Autodesk Inventor part; units mm, degrees
ref_plane "YZ Plane" through (0, 0, 0) normal (1, 0, 0) x (0, 1, 0)
ref_plane "XZ Plane" through (0, 0, 0) normal (0, 1, 0) x (-1, 0, 0)
ref_plane "XY Plane" through (0, 0, 0) normal (0, 0, 1) x (1, 0, 0)
sketch "Esquisse1" plane through (0, 0, 0) normal (0, 1, 0) x (-1, 0, 0)
  line L0 (21, 10.5) -> (-21, 10.5)
  line L1 (-21, 10.5) -> (-21, -10.5)
  line L2 (-21, -10.5) -> (21, -10.5)
  line L3 (21, -10.5) -> (21, 10.5)
  line L4 (29, 12.5) -> (-37, 12.5)
  line L5 (-37, 12.5) -> (-37, -12.5)
  line L6 (-37, -12.5) -> (29, -12.5)
  line L7 (29, -12.5) -> (29, 12.5)
  line L8 (-37, -12.5) -> (-46.0993, 12.5)
  line L9 (-46.0993, 12.5) -> (-37, 12.5)
  point P0 (0, 0)
  dimension "d0" = 20
  dimension "d1" = 42
  dimension "d2" = 21
  dimension "d3" = 10.5
  dimension "d4" = 21
  dimension "d5" = 8
  dimension "d6" = 2
  dimension "d7" = 2
  dimension "d8" = 16
extrude "Extrusion1" add sketch "Esquisse1" along normal mid plane 25
sketch "Esquisse2" plane through (37, -12.5, -12.5) normal (0.9397, 0, -0.342) x (-0.342, 0, -0.9397)
  line L0 (-26.6044, 25) -> (0, 0)
  line L1 (0, 0) -> (0, 25)
  line L2 (0, 25) -> (-26.6044, 0)
  arc A0 (-8.3022, 22.298) -> (-18.3022, 22.298) centre (-13.3022, 12.5) ccw
  line L3 (-18.3022, 22.298) -> (-8.3022, 22.298)
  line L4 (-8.3022, 22.298) -> (-8.3022, 2.702)
  line L5 (-8.3022, 2.702) -> (-18.3022, 2.702)
  line L6 (-18.3022, 2.702) -> (-18.3022, 22.298)
  arc A1 (-8.3022, 2.702) -> (-8.3022, 22.298) centre (-13.3022, 12.5) ccw
  arc A2 (-18.3022, 2.702) -> (-8.3022, 2.702) centre (-13.3022, 12.5) ccw
  arc A3 (-18.3022, 22.298) -> (-18.3022, 2.702) centre (-13.3022, 12.5) ccw
  point P0 (0.9086, 12.5)
  point P1 (-26.6044, 25)
  point P2 (-26.6044, 0)
  dimension "d11" = 22
  dimension "d13" = 10
extrude "Extrusion2" add sketch "Esquisse2" along normal blind 5 contours A3 L6 L0 | L0 L6 L2 A3 | L6 L3 L4 L2 L0 | L0 L2 L6 | L2 L6 A3 | L2 L4 L0 | L0 L4 L5 L6 L2 | A1 L2 L4 | L4 L2 A1 L0 | L0 A1 L4
sketch "Esquisse3" plane through (39.8395, -9.798, -4.6985) normal (0, -1, 0) x (0.9397, 0, -0.342)
  line L0 (5, 10) -> (0, 0)
  line L1 (0, 10) -> (5, 0)
  circle A0 centre (2.5, 5) radius 1.75
  point P0 (-39.0439, -9.2108)
  dimension "d16" = 3.5
extrude "Extrusion3" cut sketch "Esquisse3" against normal through all
sketch "Esquisse4" plane through (21, -12.5, 10.5) normal (-1, 0, 0) x (0, 0, 1)
  line L0 (-21, 3) -> (0, 3)
  line L1 (0, 3) -> (0, 6)
  line L2 (0, 6) -> (-21, 6)
  line L3 (-21, 6) -> (-21, 3)
  line L4 (-21, 0) -> (-21, 25)
  line L5 (0, 0) -> (0, 25)
  line L6 (0, 0) -> (-21, 0)
  point P0 (-10.5, 12.5)
  dimension "d19" = 3
  dimension "d20" = 3
extrude "Extrusion4" cut sketch "Esquisse4" against normal blind 7 contours L3 L2 L1 L0
sketch "Esquisse5" plane through (-21, -12.5, -10.5) normal (1, 0, 0) x (0, 0, -1)
  line L0 (-21, 6) -> (0, 6)
  line L1 (0, 6) -> (0, 3)
  line L2 (0, 3) -> (-21, 3)
  line L3 (-21, 3) -> (-21, 6)
  line L4 (-21, 25) -> (-21, 0)
  line L5 (0, 0) -> (0, 25)
  line L6 (0, 0) -> (-21, 0)
  point P0 (-10.5, 12.5)
  dimension "d23" = 3
  dimension "d24" = 3
extrude "Extrusion5" cut sketch "Esquisse5" against normal blind 7 contours L0 L1 L2 L3
sketch "Esquisse6" plane through (21, 12.5, -10.5) normal (-1, 0, 0) x (0, 0, 1)
  line L0 (21, -25) -> (0, 0)
  line L1 (0, -25) -> (21, 0)
  circle A0 centre (10.5, -12.5) radius 3
  dimension "d27" = 6
extrude "Extrusion6" cut sketch "Esquisse6" against normal through all
sketch "Esquisse7" plane through (21, 12.5, -10.5) normal (-1, 0, 0) x (0, 0, 1)
  circle A0 centre (10.5, -12.5) radius 3
  circle A1 centre (10.5, -12.5) radius 1.75
  circle A2 centre (10.5, -12.5) radius 3
  dimension "d30" = 0
  dimension "d31" = 3.5
extrude "Extrusion7" add sketch "Esquisse7" against normal blind 18
sketch "Esquisse8" plane through (21, 12.5, -10.5) normal (-1, 0, 0) x (0, 0, 1)
  circle A0 centre (10.5, -12.5) radius 4
  dimension "d34" = 8
extrude "Extrusion8" cut sketch "Esquisse8" against normal blind 3
sketch "Esquisse10" plane through (0, -12.5, 0) normal (0, -1, 0) x (1, 0, 0)
  line L0 (-21, -10.5) -> (-28, -10.5)
  line L1 (-28, -10.5) -> (-28, 10.5)
  line L2 (-28, 10.5) -> (-21, 10.5)
  line L3 (-21, 10.5) -> (-21, -10.5)
  line L4 (21, -10.5) -> (28, -10.5)
  line L5 (28, -10.5) -> (28, 10.5)
  line L6 (28, 10.5) -> (21, 10.5)
  line L7 (21, 10.5) -> (21, -10.5)
  line L8 (-28, -10.5) -> (-28, 10.5)
  line L9 (28, 10.5) -> (28, -10.5)
  line L10 (-28, -10.5) -> (-21, 0)
  line L11 (-21, 0) -> (-28, 10.5)
  line L12 (-28, 0) -> (-21, 10.5)
  line L13 (-21, -10.5) -> (-28, 0)
  line L14 (21, -10.5) -> (28, 0)
  line L15 (21, 0) -> (28, -10.5)
  line L16 (28, 10.5) -> (21, 0)
  line L17 (21, 10.5) -> (28, 0)
  circle A0 centre (-24.5, -5.25) radius 2
  circle A1 centre (24.5, -5.25) radius 2
  circle A2 centre (24.5, 5.25) radius 2
  circle A3 centre (-24.5, 5.25) radius 2
  point P0 (0, 0)
  dimension "d37" = 4
  dimension "d38" = 4
  dimension "d39" = 4
  dimension "d40" = 4
extrude "Extrusion9" cut sketch "Esquisse10" against normal through all contours A0 L10 L13 | L13 L10 A0 | A0 L13 L10 | L10 L13 A0 | A3 L12 L11 | L11 L12 A3 | A3 L11 L12 | L12 L11 A3 | A1 L15 L14 | L14 L15 A1 | L15 L14 A1 | A1 L14 L15 | A2 L17 L16 | L16 L17 A2 | L17 L16 A2 | A2 L16 L17
sketch "Esquisse11" plane through (37, 12.5, -12.5) normal (0, 0, -1) x (-1, 0, 0)
  line L0 (66, 0) -> (46, 0)
  line L1 (46, 0) -> (46, -13)
  line L2 (46, -13) -> (66, -13)
  line L3 (66, -13) -> (66, 0)
  line L4 (66, -25) -> (0, -25)
  line L5 (46, -13) -> (33, 0)
  line L6 (0, 0) -> (66, 0)
  line L7 (45, 0) -> (33, 0)
  point P0 (37, -12.5)
  dimension "d43" = 20
  dimension "d44" = 12
  dimension "d45" = 45
extrude "Extrusion10" cut sketch "Esquisse11" against normal through all
sketch "Esquisse12" plane through (-29, -12.5, 12.5) normal (0, 0, 1) x (1, 0, 0)
  line L0 (33, 25) -> (75.0993, 25)
  line L1 (75.0993, 0) -> (61.5, 0)
  line L2 (61.5, 0) -> (61.5, 25)
  line L3 (61.5, 25) -> (75.0993, 25)
  line L4 (75.0993, 25) -> (75.0993, 0)
  line L5 (57, 6) -> (57, 3)
  line L6 (66, 25) -> (66, 0)
  line L7 (61.5, 25) -> (0, 25)
  line L8 (0, 25) -> (0, 0)
  line L9 (0, 0) -> (61.5, 0)
  line L10 (61.5, 0) -> (61.5, 25)
  line L11 (75.0993, 0) -> (79.0103, 0)
  line L12 (79.0103, 0) -> (79.0103, 25)
  line L13 (79.0103, 25) -> (75.0993, 25)
  line L14 (75.0993, 25) -> (75.0993, 0)
  ellipse E0 centre (75.2481, 12.5) end of major axis (75.2481, 1.5) minor radius 3.7622 (76.9582, 2.702) -> (76.9582, 22.298) ccw
  point P0 (29, 12.5)
  dimension "d48" = 9
  dimension "d49" = 4.5
extrude "Extrusion12" cut sketch "Esquisse12" against normal through all contours L0 L6 L1 L2 | L0 L4 L1 L6 | L13 L12 L11 L4
sketch "Esquisse13" plane through (-29, -0.5, 12.5) normal (0, 0, 1) x (1, 0, 0)
  line L0 (0, -12) -> (0, 0)
  line L1 (61.5, -12) -> (0, -12)
  line L2 (0, -12) -> (0, -6)
  line L3 (0, -6) -> (61.5, -6)
  line L4 (61.5, -6) -> (61.5, -12)
  line L5 (61.5, 13) -> (0, 13)
  line L6 (0, 13) -> (0, -6)
  line L7 (0, -6) -> (61.5, -6)
  line L8 (61.5, -6) -> (61.5, 13)
  point P0 (29, 0.5)
  dimension "d54" = 6
extrude "Extrusion13" cut sketch "Esquisse13" against normal through all contours L0 L3 L4 L1
equation "\"d38\" = d37"
equation "\"d39\" = d37"
equation "\"d40\" = d37"
equation "\"d49\" = 0.5 * d48"
properties part number "forearm"
The listing builds one solid part. Answer for the finished solid, in the listing's coordinates (mm). A direction names the side the tool comes from. Coordinates: 2 decimals unless noted, no trailing zeros. Write each loop counter-clockwise with the first axis right and the second up, starting at its lowest first coordinate (ties: lowest second). Pieces come first, ordered by that corner, then holes. Notation, with made-up numbers: (31, 68) - (50, 68) arc R18 cw to (50, 85) - close; hole circle Ø11 at (60, 21.25). An arc over 180 degrees is marked (long way). One line per item, written item: value.
1) Find section D-D (z = -5.25). Give the vertices of the cut face in (x, y).
Geometry check:
outline: (-29, -6.5) - (-26.5, -6.5) - (-26.5, -0.5) - (-29, -0.5) - close; (-22.5, -6.5) - (-21, -6.5) - (-21, -0.5) - (-22.5, -0.5) - close; (21, -6.5) - (22.5, -6.5) - (22.5, 12.5) - (21, 12.5) - close; (26.5, -6.5) - (32.5, -6.5) - (32.5, 12.5) - (26.5, 12.5) - close
2) Find section C-C (y = 8). Give the vertices of the cut face in (x, z).
Geometry check:
outline: (-0.5, -12.5) - (32.5, -12.5) - (32.5, 12.5) - (-0.5, 12.5) - (-0.5, 10.5) - (21, 10.5) - (21, -10.5) - (-0.5, -10.5) - close; hole circle Ø4 at (24.5, -5.25); hole circle Ø4 at (24.5, 5.25)
3) For a pull along X with two mould halves and no side action, classify faces 1 (the flat face through (-29, -4, 0)), 2 (the flat face through (21, 5, 0)), 3 (the cylindrical face through (28.19, -0.67, 1.617)) as pulls with the +X half, pulls with the -X half, needs draft (parallel to the pull), parting line crosses it, or undercut.
Geometry check:
face 1: pulls with the -X half
face 2: undercut
face 3: needs draft
4) Find section A-A (x = -7). Give the vertices of the cut face in (y, z), and give its area (3 significant figures).
Geometry check:
outline: (-6.5, -12.5) - (1.5, -12.5) - (1.5, -10.5) - (-6.5, -10.5) - close; (-6.5, 10.5) - (1.5, 10.5) - (1.5, 12.5) - (-6.5, 12.5) - close
area: 32.0 mm2
5) Each of these flat-tipped pins is pushed along its axis until it touches: pin 1 Ø4 at (x, z) = (-17.5, 4.5) entering from +Y; pin 2 Ø6.5 at (x, z) = (-24.5, -5.25) entering from +Y; pin 3 Ø8 at (y, z) = (7.5, 3) entering from -X. Where does it stop, or does it pass through?
Geometry check:
pin 1: passes through
pin 2: stops at y = -0.5
pin 3: stops at x = 21
6) A tool of negligible diameter and unlimited length cuts with its end or side. For faces 4 (the flat face through (-23, -0.5, 0)), 5 (the flat face through (-21, -4, 0)), 6 (the flat face through (8, 1, 12.5)), 7 (the flat face through (8, -6.5, -11)), 8 (the cylindrical face through (22, 0, -4)), from which of +Z, -Z, +X, -X, +Y, -Y can it reach the whole face along a straight path? Write none if from no direction.
Geometry check:
face 4: +Z, -Z, -X, +Y
face 5: +Y, -Y
face 6: +Z, +X, -X, +Y, -Y
face 7: +Z, -Z, +X, -X, -Y
face 8: none
7) Consider line 1 along Z through (x, y) = (-24.5, -4.4); line 2 along X through (y, z) = (-3, -1.5); line 3 along Z through (x, y) = (16.5, 6). Determine where each line is inside the solid, lowest interval first. Write a range as from..to.
Geometry check:
line 1: z = -12.5..-7.25, -3.25..3.25, 7.25..12.5
line 2: x = -29..-21, 24..32.5
line 3: z = -12.5..-10.5, 10.5..12.5
8) Find section B-B (x = -24.5). Give the vertices of the cut face in (y, z), and give its area (3 significant figures).
Geometry check:
outline: (-6.5, -12.5) - (-0.5, -12.5) - (-0.5, -7.25) - (-6.5, -7.25) - close; (-6.5, -3.25) - (-0.5, -3.25) - (-0.5, 3.25) - (-6.5, 3.25) - close; (-6.5, 7.25) - (-0.5, 7.25) - (-0.5, 12.5) - (-6.5, 12.5) - close
area: 102 mm2
